The listing builds one solid part. Answer for the finished solid, in the listing's coordinates (mm). A direction names the side the tool comes from. Coordinates: 2 decimals unless noted, no trailing zeros. Write each loop counter-clockwise with the first axis right and the second up, starting at its lowest first coordinate (ties: lowest second). Pieces come first, ordered by that corner, then holes.
Autodesk Inventor part; units mm, degrees
ref_plane "YZ Plane" through (0, 0, 0) normal (1, 0, 0) x (0, 1, 0)
ref_plane "XZ Plane" through (0, 0, 0) normal (0, 1, 0) x (-1, 0, 0)
ref_plane "XY Plane" through (0, 0, 0) normal (0, 0, 1) x (1, 0, 0)
sketch "Sketch1" plane through (0, 0, 0) normal (0, 1, 0) x (-1, 0, 0)
  line L0 (0, 5) -> (0, 12)
  line L1 (0, 5) -> (7, 5)
  line L2 (7, 5) -> (7, 15)
  line L3 (7, 15) -> (0, 12)
  line L4 (0, -32.61) -> (7, -32.61)
  line L5 (7, -32.61) -> (7, -42.61)
  line L6 (0, -32.61) -> (0, -39.61)
  line L7 (0, -39.61) -> (7, -42.61)
  point P0 (0, 0)
  dimension "d2" = 5
  dimension "d3" = 7
  dimension "d5" = 7
  dimension "d6" = 10
  dimension "d7" = 7
  dimension "d8" = 10
  dimension "d9" = 7
extrude "Extrusion1" add sketch "Sketch1" along normal blind 15
sketch "Sketch2" plane through (0, 15, 0) normal (0, 1, 0) x (1, 0, 0)
  line L0 (-7, -15) -> (-7, 42.61)
  line L1 (-7, 42.61) -> (0, 39.61)
  line L2 (0, 39.61) -> (-7, 42.61)
  line L3 (0, 39.61) -> (0, -12)
  line L4 (0, -12) -> (-7, -15)
  point P0 (0, 0)
extrude "Extrusion2" add sketch "Sketch2" along normal blind 35
sketch "Sketch3" plane through (0, 50, 0) normal (0, 1, 0) x (1, 0, 0)
  line L0 (0, -12) -> (-7, -15)
  line L1 (-7, 42.61) -> (0, 39.61)
  circle A0 centre (-3.5, 31.11) radius 1.4
  circle A1 centre (-3.5, -3.5) radius 1.4
  circle A2 centre (-3.5, -3.5) radius 3.1
  circle A3 centre (-3.5, 31.11) radius 3.1
  point P0 (0, 0)
  dimension "d73" = 6.2
  dimension "d74" = 6.2
sketch "Sketch4" plane through (0, 0, 0) normal (0, -1, 0) x (1, 0, 0)
  line L0 (0, 5) -> (0, 12)
  line L1 (0, 12) -> (-7, 15)
  line L2 (-7, 15) -> (-7, 5)
  line L3 (-7, 5) -> (0, 5)
  line L4 (0, -32.61) -> (-7, -32.61)
  line L5 (-7, -32.61) -> (-7, -42.61)
  line L6 (-7, -42.61) -> (0, -39.61)
  line L7 (0, -39.61) -> (0, -32.61)
  line L8 (-7, -42.61) -> (0, -32.61)
  line L9 (0, -39.61) -> (-7, -32.61)
  line L10 (0, 5) -> (-7, 15)
  line L11 (-7, 15) -> (0, 12)
  line L12 (0, 12) -> (-7, 5)
  circle A0 centre (-2.8824, 9.1176) radius 1.4
  circle A1 centre (-2.8824, -36.7276) radius 1.4
  point P0 (0, 0)
  dimension "d14" = 2.8
  dimension "d15" = 2.8
extrude "Extrusion3" cut sketch "Sketch4" against normal blind 15 contours A0 L12 L10 | L10 L12 A0 | L12 L10 A0 | A0 L10 L12 | A1 L9 L8 | L8 L9 A1 | L9 L8 A1 | A1 L8 L9
extrude "Extrusion4" add sketch "Sketch3" along normal blind 30
sketch "Sketch6" plane through (-7, 0, -42.61) normal (-1, 0, 0) x (0, 0, 1)
  line L0 (10, 15) -> (47.61, 15)
  line L1 (28.805, 15) -> (28.805, 20)
  line L2 (28.805, 20) -> (38.805, 20)
  line L3 (38.805, 20) -> (38.805, 65)
  line L4 (38.805, 65) -> (18.805, 65)
  line L5 (18.805, 65) -> (18.805, 20)
  line L6 (18.805, 20) -> (28.805, 20)
  line L7 (18.805, 20) -> (18.805, 21.5)
  line L8 (18.805, 21.5) -> (20.305, 21.5)
  line L9 (38.805, 20) -> (38.805, 21.5)
  line L10 (38.805, 21.5) -> (37.305, 21.5)
  circle A0 centre (20.305, 21.5) radius 0.6
  circle A1 centre (37.305, 21.5) radius 0.6
  line L11 (28.805, 20) -> (28.805, 29)
  line L12 (28.805, 29) -> (28.805, 56)
  circle A2 centre (28.805, 29) radius 8.5
  circle A3 centre (28.805, 56) radius 8.5
  point P0 (42.61, 0)
  dimension "d26" = 5
  dimension "d27" = 10
  dimension "d28" = 45
  dimension "d29" = 20
  dimension "d30" = 1.5
  dimension "d31" = 1.5
  dimension "d32" = 1.5
  dimension "d33" = 1.5
  dimension "d34" = 1.2
  dimension "d35" = 1.2
  dimension "d36" = 9
  dimension "d37" = 27
  dimension "d38" = 17
  dimension "d39" = 17
extrude "Extrusion5" cut sketch "Sketch6" against normal through all contours A3 | A2 L12 L11 | L11 L12 A2
sketch "Sketch7" plane through (-7, 0, -42.61) normal (-1, 0, 0) x (0, 0, 1)
  line L0 (10, 15) -> (47.61, 15)
  line L1 (28.805, 15) -> (28.805, 20)
  line L2 (28.805, 20) -> (38.805, 20)
  line L3 (38.805, 20) -> (38.805, 65)
  line L4 (38.805, 65) -> (18.805, 65)
  line L5 (18.805, 65) -> (18.805, 20)
  line L6 (18.805, 20) -> (28.805, 20)
  line L7 (18.805, 20) -> (18.805, 21.5)
  line L8 (18.805, 21.5) -> (20.305, 21.5)
  line L9 (38.805, 20) -> (38.805, 21.5)
  line L10 (38.805, 21.5) -> (37.305, 21.5)
  circle A0 centre (20.305, 21.5) radius 0.9
  circle A1 centre (37.305, 21.5) radius 0.9
  line L11 (28.805, 20) -> (28.805, 29)
  line L12 (28.805, 29) -> (28.805, 56)
  circle A2 centre (28.805, 29) radius 8.5
  circle A3 centre (28.805, 56) radius 8.5
  point P0 (42.61, 0)
  point P1 (42.61, 0)
  dimension "d42" = 5
  dimension "d43" = 10
  dimension "d44" = 45
  dimension "d45" = 20
  dimension "d46" = 1.5
  dimension "d47" = 1.5
  dimension "d48" = 1.5
  dimension "d49" = 1.5
  dimension "d50" = 1.8
  dimension "d51" = 1.8
  dimension "d52" = 9
  dimension "d53" = 27
  dimension "d54" = 17
  dimension "d55" = 17
extrude "Extrusion6" cut sketch "Sketch7" against normal blind 5 contours A1 | A0
sketch "Sketch8" plane through (-7, 0, -42.61) normal (-1, 0, 0) x (0, 0, 1)
  circle A0 centre (20.305, 21.5) radius 0.9
  line L0 (20.305, 21.5) -> (20.305, 20)
  line L1 (20.305, 20) -> (18.805, 20)
  line L2 (18.805, 20) -> (18.805, 19)
  line L3 (18.805, 19) -> (17.805, 19)
  line L4 (17.805, 19) -> (39.805, 19)
  line L5 (39.805, 19) -> (39.805, 66)
  line L6 (39.805, 66) -> (17.805, 66)
  line L7 (17.805, 66) -> (17.805, 19)
  point P0 (42.61, 0)
  dimension "d58" = 1.5
  dimension "d59" = 1.5
  dimension "d60" = 1
  dimension "d61" = 1
  dimension "d62" = 22
  dimension "d63" = 47
extrude "Extrusion7" cut sketch "Sketch8" against normal blind 2
sketch "Sketch9" plane through (-7, 0, -42.61) normal (-1, 0, 0) x (0, 0, 1)
  line L0 (10, 0) -> (0, 0)
  line L1 (0, 0) -> (0, 10)
  line L2 (0, 10) -> (10, 10)
  line L3 (10, 10) -> (10, 0)
  line L4 (47.61, 0) -> (57.61, 0)
  line L5 (57.61, 0) -> (57.61, 10)
  line L6 (57.61, 10) -> (47.61, 10)
  line L7 (47.61, 10) -> (47.61, 0)
  line L8 (57.61, 0) -> (47.61, 0)
  point P0 (42.61, 0)
  dimension "d66" = 10
  dimension "d67" = 10
extrude "Extrusion8" add sketch "Sketch9" along normal blind 40
chamfer "Chamfer1" distance 2 angle 45 8 edges at (-47, 5, -42.61) (-47, 0, -37.61) (-47, 5, -32.61) (-47, 10, -37.61) (-47, 0, 10) (-47, 5, 15) (-47, 5, 5) (-47, 10, 10)
properties part number "Back Support" material "ABS Plastic"
Q1. Find the intervals of material crossed by probe 1 along Z at (x, y) = (-3.5, 73.25); probe 2 along X at (y, z) = (61, -31); probe 3 along Z at (x, y) = (-24, 8), in increasing order.
Answers below:
probe 1: z = -34.21 to -32.51, -29.71 to -28.01, 0.4 to 2.1, 4.9 to 6.6
probe 2: x = -6.6 to -4.9, -2.1 to -0.4
probe 3: z = -42.61 to -32.61, 5 to 15
Q2. The part is cut by section A-A, the plane x = -13. Write down the section's boundary in (y, z).
Answers below:
outline: (0, -42.61) - (10, -42.61) - (10, -32.61) - (0, -32.61) - close; (0, 5) - (10, 5) - (10, 15) - (0, 15) - close
Q3. The part is cut by section D-D, the plane y = 39. Write down the section's boundary in (x, z) (3 decimals), then the cut area to 3 significant figures.
Answers below:
outline: (-7, -42.61) - (0, -39.61) - (0, 12) - (-7, 15) - (-7, -2.805) - (-5, -2.805) - (-5, -24.805) - (-7, -24.805) - close
area: 338 mm2
Q4. Which of the six approach directions +Z, -Z, +X, -X, +Y, -Y give full straight-line access (tool end or side, diameter ignored) to faces 4 (the face through (-4, 50, 3)), 5 (the face through (-2.13, 7.395, -35.547)), 6 (the face through (-22, 6, -32.61))?
Answers below:
face 4: +Y
face 5: -Y
face 6: +X, -X, -Y
Q5. Given pin 1 (11 mm diameter, centred on x = -33.5, z = 9.5, fed in from +Y); pin 2 (0.9 mm diameter, centred on y = 21, z = -22.5, fed in from -X); pin 3 (1.6 mm diameter, centred on x = -6, y = 40.5, fed in from +Z); pin 4 (3 mm diameter, centred on x = -3, z = -36.5, fed in from -Y), each flat-ended and moving along its own axis, determine where each tip first touches the part or whether it passes through.
Answers below:
pin 1: stops at y = 10
pin 2: stops at x = -5
pin 3: stops at z = 14.91
pin 4: stops at y = 0
Q6. The part is cut by section B-B, the plane y = 65. Write down the section's boundary in (x, z).
Answers below:
outline: circle Ø6.2 at (-3.5, -31.11); circle Ø6.2 at (-3.5, 3.5); hole circle Ø2.8 at (-3.5, -31.11); hole circle Ø2.8 at (-3.5, 3.5)
Q7. Determine the mould class of faces 1 (the face through (-3.5, 24.6, 13.5)), 2 (the face through (-22, 6, 5)), 3 (the face through (-2, 80, -30)) for opening direction Z: released by +Z, released by -Z, zero draft, split by the parting line, or undercut.
Answers below:
face 1: released by +Z
face 2: undercut
face 3: zero draft
Q8. The part is cut by section C-C, the plane z = -31.11. Write down the section's boundary in (x, y).
Answers below:
outline: (-7, 15) - (0, 15) - (0, 50) - (-0.4, 50) - (-0.4, 80) - (-2.1, 80) - (-2.1, 50) - (-4.9, 50) - (-4.9, 80) - (-6.6, 80) - (-6.6, 50) - (-7, 50) - close
